Geometry: see drawing. Coordinates: mm, zero at the bounding-box minimum. Round coordinates to 2 decimals unless told otherwise and drop trailing zeros. Loops run counter-clockwise (first coordinate to the right, second up) from the corner with the lowest first, then second, coordinate; pieces in that order, holes last. Notation, with made-up numbers: (5.25, 88.25) -> (20.25, 88.25) arc R26 ccw to (20.25, 102.25) -> close; hole circle Ø1 at (52.5, -23.75). An arc over 180 degrees is marked (long way). Write item = value, one per line.
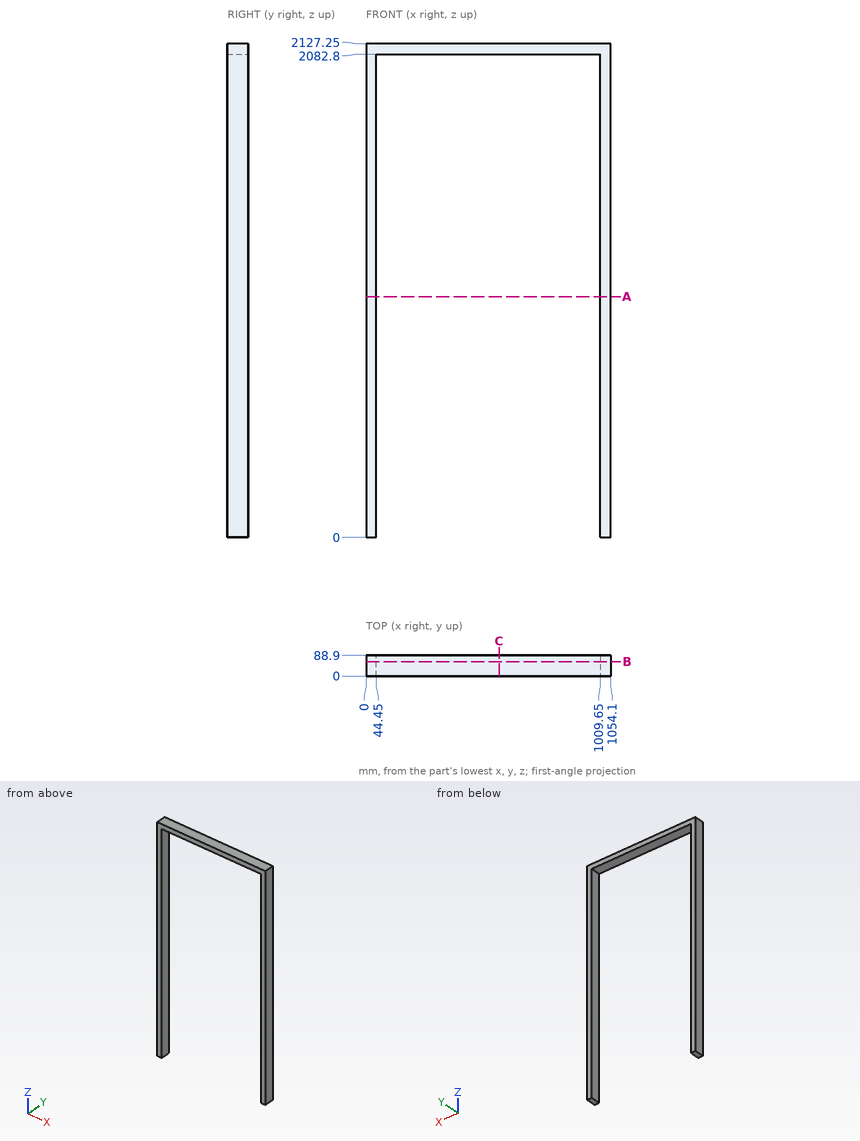
1. Section query A-A (z = 1038.5). Return the cut outline in (x, y), then the cut area to 3 significant figures.
Evaluation:
outline = (0, 0) -> (44.45, 0) -> (44.45, 88.9) -> (0, 88.9) -> close; (1009.65, 0) -> (1054.1, 0) -> (1054.1, 88.9) -> (1009.65, 88.9) -> close
area = 7,900 mm²
2. Line query: probe 1 along X at (y, z) = (66.5, 1745); probe 2 along Z at (x, y) = (540.5, 79). Output: solid intervals per line, ascending. Write a range as from..to.
Evaluation:
probe_1 = 0..44.45, 1009.65..1054.1
probe_2 = 2082.8..2127.25
3. Section query C-C (x = 574). Return the cut outline in (y, z).
Evaluation:
outline = (0, 2082.8) -> (88.9, 2082.8) -> (88.9, 2127.25) -> (0, 2127.25) -> close
4. Section query B-B (y = 62). Return the cut outline in (x, z), then the cut area to 3 significant figures.
Evaluation:
outline = (0, 0) -> (44.45, 0) -> (44.45, 2082.8) -> (1009.65, 2082.8) -> (1009.65, 0) -> (1054.1, 0) -> (1054.1, 2127.25) -> (0, 2127.25) -> close
area = 232,000 mm²
